Geometry check sheet. Reference: the model listing, model coordinates, mm. Face numbers are marked on the shaded views. A direction names the side the tool comes from. Give positions to 0.01 mm unless a question says otherwise; leave off trailing zeros. Write each loop counter-clockwise with the first axis right and the second up, starting at its lowest first coordinate (ties: lowest second). Pieces come first, ordered by that corner, then holes. Notation, with made-up numbers: (-35, 53.25) - (-12, 53.25) arc R32 ccw to (-12, 79.25) - close; hole circle Ø4 at (-25, 51.5). An arc over 180 degrees is marked (long way). Use a Markdown table: item, result.
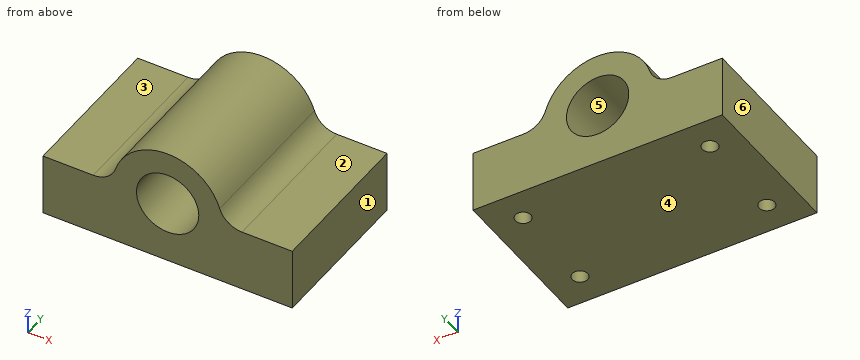
```python
from build123d import *

# Parameters (mm, degrees)
F1_DEPTH = 127
F2_R     = 6.35
F3_DEPTH = 31.75


with BuildPart() as f1:
    # F0 (on Front) → F1 (new body)
    with BuildSketch(Plane.XZ):
        with BuildLine():
            ThreePointArc((60.634122, 0), (49.361852, 3.692968), (42.459989, 13.34006))
            ThreePointArc((42.459989, 13.34006), (0, 44.506268), (-42.459989, 13.34006))
            ThreePointArc((-42.459989, 13.34006), (-49.361852, 3.692968), (-60.634122, 0))
            Line((-60.634122, 0), (-101.6, 0))
            Line((-101.6, 0), (-101.6, -50.8))
            Line((-101.6, -50.8), (101.6, -50.8))
            Line((101.6, -50.8), (101.6, 0))
            Line((101.6, 0), (60.634122, 0))
        make_face()
        with BuildLine():
            ThreePointArc((-25.4, 0), (0, 25.4), (25.4, 0))
            ThreePointArc((25.4, 0), (0, -25.4), (-25.4, 0))
        make_face(mode=Mode.SUBTRACT)
    extrude(amount=F1_DEPTH)

    # F2 (on face) → F3 (cut)
    with BuildSketch(Plane(origin=(0, 0, -50.8), x_dir=(1, 0, 0), z_dir=(0, 0, -1))):
        with Locations((-76.2, 101.6)):
            Circle(F2_R)
        with Locations((-76.2, 25.4)):
            Circle(F2_R)
        with Locations((76.2, 25.4)):
            Circle(F2_R)
        with Locations((76.2, 101.6)):
            Circle(F2_R)
    extrude(amount=-F3_DEPTH, mode=Mode.SUBTRACT)


solid = f1.part
```
1) Section check B-B on z = -27.5. Record the boundary of the cut face in (x, y).
Working result:
| item | result |
|---|---|
| outline | (-101.6, -127) - (101.6, -127) - (101.6, 0) - (-101.6, 0) - close; hole circle Ø12.7 at (-76.2, -101.6); hole circle Ø12.7 at (-76.2, -25.4); hole circle Ø12.7 at (76.2, -101.6); hole circle Ø12.7 at (76.2, -25.4) |
2) Section check A-A on x = 0. Record the boundary of the cut face in (y, z).
Working result:
| item | result |
|---|---|
| outline | (-127, -50.8) - (0, -50.8) - (0, -25.4) - (-127, -25.4) - close; (-127, 25.4) - (0, 25.4) - (0, 44.51) - (-127, 44.51) - close |
3) Mould release check, pull along X, two halves, no side actions. Record for the marked faces 4, 5 and 6: pulls with the +X half, pulls with the -X half, needs draft (parallel to the pull), parting line crosses it, or undercut.
Working result:
| item | result |
|---|---|
| face 4 | needs draft |
| face 5 | undercut |
| face 6 | pulls with the -X half |
4) Section check D-D on z = -14.5. Record the boundary of the cut face in (x, y), then the cut area to 3 significant figures.
Working result:
| item | result |
|---|---|
| outline | (-101.6, -127) - (-20.85, -127) - (-20.85, 0) - (-101.6, 0) - close; (20.85, -127) - (101.6, -127) - (101.6, 0) - (20.85, 0) - close |
| area | 20,500 mm² |
5) Depth check by flat-ended pin: P1, Ø6.5, axis at x = 74, y = -102.5, coming from the -Z side; P2, Ø16.5, axis at x = -76.2, y = -25.4, coming from the +Z side; P3, Ø1.5, axis at y = -23.5, z = 6, coming from the -X side. Enter the tip coordinate at first touch or a pass-through.
Working result:
| item | result |
|---|---|
| P1 | stops at z = -19.05 |
| P2 | stops at z = 0 |
| P3 | stops at x = -47.5 |
6) Set-up check for the marked faces 1, 2 and 3: record each of +Z, -Z, +X, -X, +Y, -Y from which the full face is reachable in a straight line by a thin tool's end or side.
Working result:
| item | result |
|---|---|
| face 1 | +Z, -Z, +X, +Y, -Y |
| face 2 | +Z, +X, +Y, -Y |
| face 3 | +Z, -X, +Y, -Y |
7) Material ranges on L1, parallel to X at y = -25.4, z = -36.5; L2, parallel to Y at x = -76.2, z = -30; L3, parallel to Z at x = 0, y = -69, recorded low to high. Write a range as from..to.
Working result:
| item | result |
|---|---|
| L1 | x = -101.6..-82.55, -69.85..69.85, 82.55..101.6 |
| L2 | y = -127..-107.95, -95.25..-31.75, -19.05..0 |
| L3 | z = -50.8..-25.4, 25.4..44.51 |
8) Section check C-C on y = -101.6. Record the boundary of the cut face in (x, z).
Working result:
| item | result |
|---|---|
| outline | (-101.6, -50.8) - (-82.55, -50.8) - (-82.55, -19.05) - (-69.85, -19.05) - (-69.85, -50.8) - (69.85, -50.8) - (69.85, -19.05) - (82.55, -19.05) - (82.55, -50.8) - (101.6, -50.8) - (101.6, 0) - (60.63, 0) arc R19.05 cw to (42.46, 13.34) arc R44.51 ccw to (-42.46, 13.34) arc R19.05 cw to (-60.63, 0) - (-101.6, 0) - close; hole circle Ø50.8 at (0, 0) |
